```python
from build123d import *

# Parameters (mm, degrees)
IZIM1_W                     = 80
IZIM1_H                     = 80
Y_KSEKLIK_EKSTR_ZYON1_DEPTH = 65
IZIM3_W                     = 45
IZIM3_H                     = 50
KES_EKSTR_ZYON1_DEPTH       = 40
IZIM4_W                     = 20
IZIM4_H                     = 46
KES_EKSTR_ZYON2_DEPTH       = 80
IZIM5_W                     = 25
IZIM5_H                     = 20
KES_EKSTR_ZYON3_DEPTH       = 111.566721937


with BuildPart() as part:
    # Çizim1 → Yükseklik-Ekstrüzyon1 (new body)
    with BuildSketch(Plane.XY):
        Rectangle(IZIM1_W, IZIM1_H)
    extrude(amount=Y_KSEKLIK_EKSTR_ZYON1_DEPTH)

    # Çizim3 → Kes-Ekstrüzyon1 (cut)
    with BuildSketch(Plane.XY.offset(65)):
        Rectangle(IZIM3_W, IZIM3_H)
    extrude(amount=-KES_EKSTR_ZYON1_DEPTH, mode=Mode.SUBTRACT)

    # Çizim4 → Kes-Ekstrüzyon2 (cut)
    with BuildSketch(Plane(origin=(40, 0, 0), x_dir=(0, 0, -1), z_dir=(1, 0, 0))):
        with Locations((-35, 3)):
            Rectangle(IZIM4_W, IZIM4_H)
    extrude(amount=-KES_EKSTR_ZYON2_DEPTH, mode=Mode.SUBTRACT)

    # Çizim5 → Kes-Ekstrüzyon3 (cut, through all)
    with BuildSketch(Plane.XZ.offset(40)):
        with Locations((27.5, 55)):
            Rectangle(IZIM5_W, IZIM5_H)
    extrude(amount=-KES_EKSTR_ZYON3_DEPTH, mode=Mode.SUBTRACT)


solid = part.part
```
Verification items for the finished model (mm, model axes). A direction names the side the tool comes from. Coordinates: 2 decimals unless noted, no trailing zeros. Order: outer loops, then holes, each group sorted by start corner. A loop starts at its lowest first (then second) coordinate and runs counter-clockwise, first axis right, second up. Notation, with made-up numbers: (-7.5, -38.5) -> (46.5, -38.5) arc R18 ccw to (46.5, -26.5) -> close; hole circle Ø3 at (20, 49). An arc over 180 degrees is marked (long way). Answer as CSV lines item,"result". Start each with the question number.
1) Cross-section at B-B, the plane z = 31. Record the boundary of the cut face in (x, y).
2) Cross-section at A-A, the plane y = 10.5. Record the boundary of the cut face in (x, z), then the cut area to 3 significant figures.
3) Gauge pin test, flat ends, axial feed: pin 1 Ø12 at (y, z) = (-32.5, 56.5) entering from +X; pin 2 Ø3 at (y, z) = (7.5, 46.5) entering from +X; pin 3 Ø6 at (x, y) = (22.5, -27) entering from +Z. Record the tip position at first contact, or that the pin passes through.
4) Release check for a two-part mould opening along Y. For faces 1 (the face through (40, -1, 17)), 2 (the face through (-1, -40, 32)), 3 (the face through (-4, 25, 55)), 4 (the face through (31, -20, 35)) record: released by +Y, released by -Y, zero draft, split by the parting line, or undercut.
5) Cross-section at C-C, the plane x = -5.5. Record the boundary of the cut face in (y, z).
6) Material ranges on L1, parallel to Z at x = -24, y = 0; L2, parallel to Y at x = 10.5, z = 49.5; L3, parallel to Y at x = 15, z = 31, recorded low to high. Write a range as [from, to].
7) Set-up check for faces 5 (the face through (22.5, -23, 35)), 6 (the face through (1, 26, 35)), 7 (the face through (27, -30, 45)): record each of +Z, -Z, +X, -X, +Y, -Y from which the full face is reachable in a straight line by a thin tool's end or side.
8) Cross-section at D-D, the plane y = -32. Record the boundary of the cut face in (x, z).
Conclusion:
1,outline,"(-40, -40) -> (40, -40) -> (40, -20) -> (22.5, -20) -> (22.5, -25) -> (-22.5, -25) -> (-22.5, -20) -> (-40, -20) -> close; (-40, 26) -> (40, 26) -> (40, 40) -> (-40, 40) -> close"
2,outline,"(-40, 0) -> (40, 0) -> (40, 25) -> (-40, 25) -> close; (-40, 45) -> (-22.5, 45) -> (-22.5, 65) -> (-40, 65) -> close"
2,area,"2,350 mm²"
3,pin 1,"stops at x = 15"
3,pin 2,"stops at x = -22.5"
3,pin 3,"stops at z = 45"
4,face 1,"zero draft"
4,face 2,"released by -Y"
4,face 3,"undercut"
4,face 4,"undercut"
5,outline,"(-40, 0) -> (40, 0) -> (40, 65) -> (25, 65) -> (25, 45) -> (26, 45) -> (26, 25) -> (-25, 25) -> (-25, 65) -> (-40, 65) -> close"
6,L1,"z = [0, 25], [45, 65]"
6,L2,"y = [-40, -25], [25, 40]"
6,L3,"y = [-40, -25], [26, 40]"
7,face 5,"+Z"
7,face 6,"+X, -X"
7,face 7,"+Z, +X, +Y, -Y"
8,outline,"(-40, 0) -> (40, 0) -> (40, 45) -> (15, 45) -> (15, 65) -> (-40, 65) -> close"
